Read the model definition and answer for the solid it produces. Units are mm, in the model's axes. Face numbers are marked on the shaded views. A direction names the side the tool comes from. Coordinates: 2 decimals unless noted, no trailing zeros. Order: outer loops, then holes, each group sorted by start corner. A loop starts at its lowest first (then second) coordinate and runs counter-clockwise, first axis right, second up. Notation, with made-up numbers: M -18,-18.75 L 19,-18.75 A31 cw 19,15.25 Z; hole C -1.5,63 d9. An arc over 180 degrees is marked long. One line per question, with ' | ' between items. Start each with the question number.
1) A tool of negligible diameter and unlimited length cuts with its end or side. For the marked faces 1 and 2, from which of +Z, -Z, +X, -X, +Y, -Y can it reach the whole face along a straight path? Write none if from no direction.
2) Find section A-A, the plane y = 17.5. Write down the section's boundary in (x, z), plus the area to 3 significant figures.
3) Find section C-C, the plane x = -3.5. Write down the section's boundary in (y, z), plus the area to 3 significant figures.
4) Find section B-B, the plane y = 11. Write down the section's boundary in (x, z) (3 decimals), plus the area to 3 significant figures.
5) The mould has two halves that part along Z. Classify the marked faces 3, 4, 5 and 6: +Z half, -Z half, draft (parallel to the pull), parting line (faces both ways), or undercut.
6) Given P1, Ø4, axis at x = 11, y = 0, coming from the -Z side; P2, Ø1.5, axis at x = 7.78, y = 7.78, coming from the -Z side; P3, Ø4, axis at x = 10.5, z = 43.5, coming from the -Y side; P4, Ø10, axis at x = -11, z = 7, coming from the -Y side, each flat-ended and moving along its own axis, determine where each tip first touches the part or whether it passes through.
7) Consider probe 1 along X at (y, z) = (0, 3) (3 decimals); probe 2 along Z at (x, y) = (5.75, 21.5); probe 3 along Y at (x, z) = (-8.75, 57). Determine where each line is inside the solid, lowest interval first.
8) Find section D-D, the plane z = 36.5. Write down the section's boundary in (x, y), plus the area to 3 significant figures.
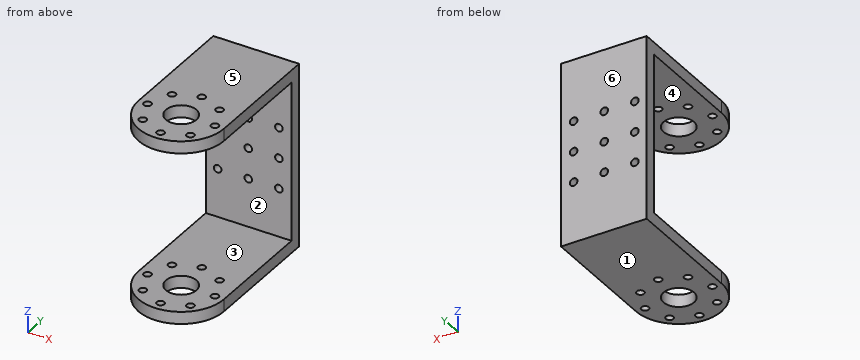
from build123d import *

# Parameters (mm, degrees)
SKETCH_2_R          = 5
SKETCH_2_R_2        = 1.225
EXTRUDE_1_DEPTH     = 60
SKETCH_9_W          = 52
SKETCH_9_H          = 50
CUT_EXTRUDE_1_DEPTH = 60
SKETCH_11_R         = 1.25
CUT_EXTRUDE_3_DEPTH = 60


with BuildPart() as part:
    # 스케치2 → 보스-돌출1 (new body)
    with BuildSketch(Plane.XY):
        with BuildLine():
            Line((-14, 0), (-14, 40))
            Line((-14, 40), (14, 40))
            Line((14, 40), (14, 0))
            ThreePointArc((14, 0), (0, -14), (-14, 0))
        make_face()
        Circle(SKETCH_2_R, mode=Mode.SUBTRACT)
        with Locations((0, 11)):
            Circle(SKETCH_2_R_2, mode=Mode.SUBTRACT)
        with Locations((7.778174593, 7.778174593)):
            Circle(SKETCH_2_R_2, mode=Mode.SUBTRACT)
        with Locations((11, 0)):
            Circle(SKETCH_2_R_2, mode=Mode.SUBTRACT)
        with Locations((7.778174593, -7.778174593)):
            Circle(SKETCH_2_R_2, mode=Mode.SUBTRACT)
        with Locations((0, -11)):
            Circle(SKETCH_2_R_2, mode=Mode.SUBTRACT)
        with Locations((-7.778174593, -7.778174593)):
            Circle(SKETCH_2_R_2, mode=Mode.SUBTRACT)
        with Locations((-11, 0)):
            Circle(SKETCH_2_R_2, mode=Mode.SUBTRACT)
        with Locations((-7.778174593, 7.778174593)):
            Circle(SKETCH_2_R_2, mode=Mode.SUBTRACT)
    extrude(amount=EXTRUDE_1_DEPTH)

    # 스케치9 → 컷-돌출1 (cut)
    with BuildSketch(Plane(origin=(14, 0, 0), x_dir=(0, 0, -1), z_dir=(1, 0, 0))):
        with Locations((-30, 11)):
            Rectangle(SKETCH_9_W, SKETCH_9_H)
    extrude(amount=-CUT_EXTRUDE_1_DEPTH, mode=Mode.SUBTRACT)

    # 스케치11 → 컷-돌출3 (cut)
    with BuildSketch(Plane(origin=(0, 40, 0), x_dir=(1, 0, 0), z_dir=(0, 1, 0))):
        with Locations(Location((-10.142727679, -39.786307008, 0), (0, 0, 270))):
            Circle(SKETCH_11_R)
        with Locations(Location((-10.142727679, -19.786307008, 0), (0, 0, 270))):
            Circle(SKETCH_11_R)
        with Locations(Location((-10.142727679, -29.786307008, 0), (0, 0, 270))):
            Circle(SKETCH_11_R)
        with Locations(Location((-0.142727679, -39.786307008, 0), (0, 0, 270))):
            Circle(SKETCH_11_R)
        with Locations(Location((-0.142727679, -29.786307008, 0), (0, 0, 270))):
            Circle(SKETCH_11_R)
        with Locations(Location((-0.142727679, -19.786307008, 0), (0, 0, 270))):
            Circle(SKETCH_11_R)
        with Locations(Location((9.857272321, -19.786307008, 0), (0, 0, 270))):
            Circle(SKETCH_11_R)
        with Locations(Location((9.857272321, -29.786307008, 0), (0, 0, 270))):
            Circle(SKETCH_11_R)
        with Locations(Location((9.857272321, -39.786307008, 0), (0, 0, 270))):
            Circle(SKETCH_11_R)
    extrude(amount=-CUT_EXTRUDE_3_DEPTH, mode=Mode.SUBTRACT)


solid = part.part
Report:
1) face 1: -Z, +X, -X, +Y, -Y | face 2: +X, -X, -Y
2) outline: M -14,0 L 14,0 L 14,4 L -14,4 Z; M -14,56 L 14,56 L 14,60 L -14,60 Z | area: 224 mm^2
3) outline: M -13.56,0 L -3.57,0 L -3.57,4 L -13.56,4 Z; M -13.56,56 L -3.57,56 L -3.57,60 L -13.56,60 Z; M 3.57,0 L 40,0 L 40,60 L 3.57,60 L 3.57,56 L 36,56 L 36,4 L 3.57,4 Z | area: 579 mm^2
4) outline: M -14,0 L -1.225,0 L -1.225,4 L -14,4 Z; M -14,56 L -1.225,56 L -1.225,60 L -14,60 Z; M 1.225,0 L 14,0 L 14,4 L 1.225,4 Z; M 1.225,56 L 14,56 L 14,60 L 1.225,60 Z | area: 204 mm^2
5) face 3: undercut | face 4: undercut | face 5: +Z half | face 6: draft
6) P1: stops at z = 0 | P2: passes through | P3: stops at y = 36 | P4: stops at y = -12.12
7) probe 1: x = -14 to -12.225, -9.775 to -5, 5 to 9.775, 12.225 to 14 | probe 2: z = 0 to 4, 56 to 60 | probe 3: y = -10.93 to -8.52, -7.03 to 7.03, 8.52 to 40
8) outline: M -14,36 L 14,36 L 14,40 L -14,40 Z | area: 112 mm^2
